Geometry: see drawing. Coordinates: mm, zero at the bounding-box minimum. Coordinates: 2 decimals unless noted, no trailing zeros. Write each loop counter-clockwise with the first axis right and the second up, starting at its lowest first coordinate (ties: lowest second). Pieces come first, ordered by that corner, then holes. Notation, with made-up numbers: (38.25, 84) - (72.25, 84) arc R23 ccw to (72.25, 100) - close; hole circle Ø8 at (-19, -20). An arc over 180 degrees is marked (long way). One line per question, with ' | ' between items. Start each with the question number.
1) Draft query along X for the marked faces 1 and 2. Return one class per face: released by +X, released by -X, zero draft, split by the parting line, or undercut.
2) Line query: line 1 (Y direction, x = 88.5, z = 12.5); line 2 (Z direction, x = 810, y = 173); line 3 (Y direction, x = 636, z = 24.5) (1 decimal). Output: solid intervals per line, ascending.
3) First-contact query: P1, Ø5, axis at x = 528, y = 233, coming from the -Z side; P2, Ø10.5, axis at y = 465, z = 9, coming from the -X side; P3, Ø3, axis at x = 665.5, z = 35.5, coming from the -Y side (1 decimal); P4, Ø10, axis at x = 246.5, z = 49, coming from the +Y side (1 decimal). Flat tips, straight axial feed; report the tip coordinate or a pass-through.
4) Section query D-D on x = 248.5. Return loops of the section in (y, z).
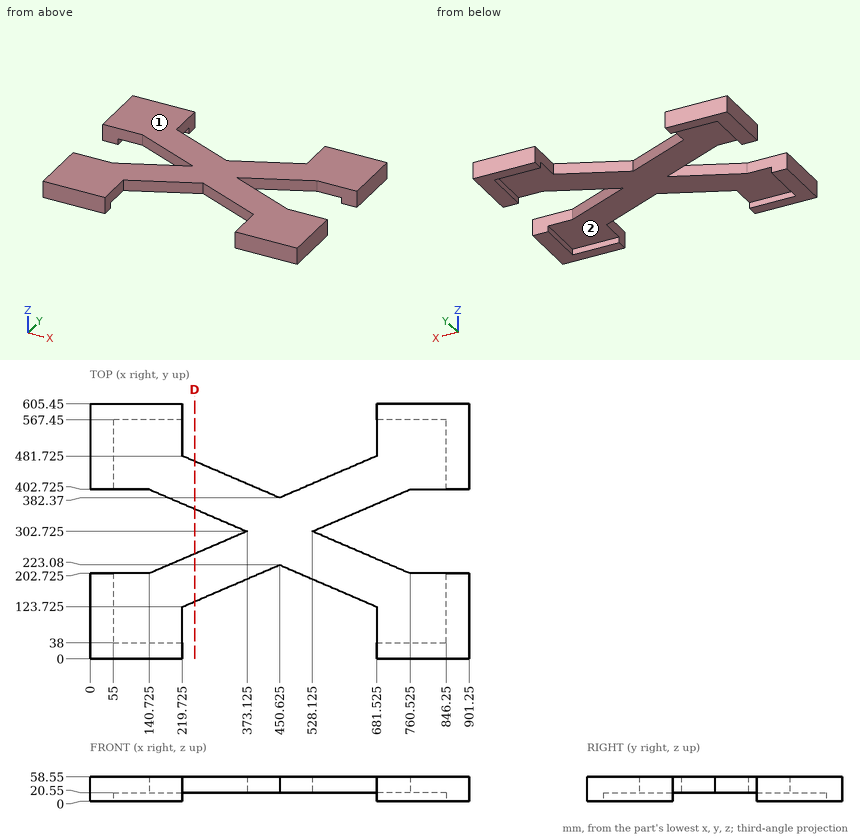
Answer key:
1) face 1: zero draft | face 2: undercut
2) line 1: 0 to 38, 567.45 to 605.45 | line 2: 20.55 to 58.55 | line 3: 143.3 to 256.3, 349.1 to 462.1
3) P1: z = 20.55 | P2: x = 0 | P3: y = 130 | P4: y = 472.4
4) outline: (136.11, 20.55) - (249.1, 20.55) - (249.1, 58.55) - (136.11, 58.55) - close; (356.35, 20.55) - (469.34, 20.55) - (469.34, 58.55) - (356.35, 58.55) - close
